Geometry: final body of the model. Coordinates: model frame, mm. A direction names the side the tool comes from. Give positions to 0.01 mm unless a question says otherwise; leave off trailing zeros. Loops run counter-clockwise (first coordinate to the right, second up) from the corner with the lowest first, then second, coordinate; pieces in that order, holes last.
```python
from build123d import *

# Parameters (mm, degrees)
SKETCH1_R      = 2.5
SKETCH1_R_2    = 6.85
EXTRUDE1_DEPTH = 100


with BuildPart() as part:
    # Sketch1 → Extrude1 (new body)
    with BuildSketch(Plane.XY):
        Polygon((-20, -4), (-16, -4), (-16, -11), (-13.828427, -11), (-10, -7.171573), (-10, 7.171573), (-13.828427, 11), (-16, 11), (-16, 4), (-20, 4), (-20, 20), (-4, 20), (-4, 16), (-11, 16), (-11, 13.828427), (-7.171573, 10), (7.171573, 10), (11, 13.828427), (11, 16), (4, 16), (4, 20), (20, 20), (20, 4), (16, 4), (16, 11), (13.828427, 11), (10, 7.171573), (10, -7.171573), (13.828427, -11), (16, -11), (16, -4), (20, -4), (20, -20), (4, -20), (4, -16), (11, -16), (11, -13.828427), (7.171573, -10), (-7.171573, -10), (-11, -13.828427), (-11, -16), (-4, -16), (-4, -20), (-20, -20), align=None)
        with Locations((-15.5, -15.5)):
            Circle(SKETCH1_R, mode=Mode.SUBTRACT)
        with Locations((-15.5, 15.5)):
            Circle(SKETCH1_R, mode=Mode.SUBTRACT)
        with Locations((15.5, -15.5)):
            Circle(SKETCH1_R, mode=Mode.SUBTRACT)
        with Locations((15.5, 15.5)):
            Circle(SKETCH1_R, mode=Mode.SUBTRACT)
        Circle(SKETCH1_R_2, mode=Mode.SUBTRACT)
    extrude(amount=-EXTRUDE1_DEPTH)


solid = part.part
```
Q1. Reachability of faces 1 (the face through (11.89, -9.06, -49.3)), 2 (the face through (18, -4, -49)), 3 (the face through (-18, 4, -49)) from +Z, -Z, +X, -X, +Y, -Y: full face, straight path, thin tool, end or side. Return the list, or none.
Q2. Mould query, pull axis X, two halves, no side actions, for faces 4 (the face through (12, 20, -49)), 5 (the face through (-10, 0, -49)), 6 (the face through (20, -12, -49)). Classes: +X half, -X half, draft (parallel to the pull), parting line (faces both ways), or undercut.
Q3. Section query D-D, the plane x = -15. Return loops of the section in (y, z), and give its area (3 significant figures).
Q4. Material intervals for probe 1 along X at (y, z) = (-7, -71); probe 2 along Y at (x, z) = (-15.5, -23.5); probe 3 along X at (y, z) = (5, -24), sorted ascending.
Q5. Section query A-A, the plane y = 0. Return loops of the section in (x, z).
Q6. Pin query (flat end, axial travel): pin 1 Ø6 at (y, z) = (0, -13) entering from +X. Return the tip coordinate at first contact, or that it passes through.
Q7. Section query C-C, the plane z = -19. State how many separate pieces and enclosed holes the cut face has, and give its area (3 significant figures).
Resolved:
1. face 1: +Z, -Z
1. face 2: +Z, -Z, +X
1. face 3: +Z, -Z, -X
2. face 4: draft
2. face 5: undercut
2. face 6: +X half
3. outline: (-20, -100) - (-17.95, -100) - (-17.95, 0) - (-20, 0) - close; (-13.05, -100) - (-11, -100) - (-11, 0) - (-13.05, 0) - close; (11, -100) - (13.05, -100) - (13.05, 0) - (11, 0) - close; (17.95, -100) - (20, -100) - (20, 0) - (17.95, 0) - close
3. area: 820 mm2
4. probe 1: x = -20 to -16, -10 to 10, 16 to 20
4. probe 2: y = -20 to -18, -13 to -11, 11 to 13, 18 to 20
4. probe 3: x = -20 to -16, -10 to -4.68, 4.68 to 10, 16 to 20
5. outline: (-10, -100) - (-6.85, -100) - (-6.85, 0) - (-10, 0) - close; (6.85, -100) - (10, -100) - (10, 0) - (6.85, 0) - close
6. pin 1: stops at x = 10
7. separate pieces: 1
7. enclosed holes: 5
7. area: 777 mm2
